Here's how the part is built. I have some questions about the finished solid (model axes, mm). A direction names the side the tool comes from. Round coordinates to 2 decimals unless told otherwise and drop trailing zeros. Loops run counter-clockwise (first coordinate to the right, second up) from the corner with the lowest first, then second, coordinate; pieces in that order, holes last. Notation, with made-up numbers: M 75,58 L 84,58 A22 ccw 84,95 Z; hole C 72,29 d4. An arc over 180 degrees is marked long. Use a Markdown table: item, result.
```python
from build123d import *

# Parameters (mm, degrees)
SKETCH1_W           = 100
SKETCH1_H           = 48
BOSS_EXTRUDE1_DEPTH = 7
CUT_EXTRUDE1_REACH  = 113.144
SKETCH2_R           = 4.5
SKETCH2_R_2         = 2.2
SKETCH3_W           = 100
SKETCH3_H           = 8
BOSS_EXTRUDE2_DEPTH = 10.2
SKETCH4_R           = 6.6
CUT_EXTRUDE2_DEPTH  = 5.25
SKETCH5_R           = 2.6
CUT_EXTRUDE3_DEPTH  = 7
SKETCH7_R           = 1.5
CUT_EXTRUDE4_DEPTH  = 112.391382072
CUT_EXTRUDE5_REACH  = 114.249
SKETCH8_R           = 1.7
SKETCH9_R           = 3
CUT_EXTRUDE6_DEPTH  = 3.5
BOSS_EXTRUDE3_DEPTH = 7
CUT_EXTRUDE7_REACH  = 116.246
FILLET1_R           = 10
FILLET2_R           = 10


with BuildPart() as part:
    # Sketch1 → Boss-Extrude1 (new body)
    with BuildSketch(Plane.XY):
        with Locations((50, 24)):
            Rectangle(SKETCH1_W, SKETCH1_H)
    extrude(amount=BOSS_EXTRUDE1_DEPTH)

    # Sketch2 → Cut-Extrude1 (cut, up to next)
    with BuildSketch(Plane.XY.offset(7), mode=Mode.PRIVATE) as cut_extrude1_sk1:
        with Locations((15, 29)):
            Circle(SKETCH2_R)
    cut_extrude1_tool1 = extrude(cut_extrude1_sk1.sketch, amount=-CUT_EXTRUDE1_REACH, mode=Mode.PRIVATE) & part.part
    # Sketch2 → Cut-Extrude1 (cut, up to next)
    with BuildSketch(Plane.XY.offset(7), mode=Mode.PRIVATE) as cut_extrude1_sk2:
        with Locations((33.75, 29)):
            Circle(SKETCH2_R_2)
    cut_extrude1_tool2 = extrude(cut_extrude1_sk2.sketch, amount=-CUT_EXTRUDE1_REACH, mode=Mode.PRIVATE) & part.part
    # Sketch2 → Cut-Extrude1 (cut, up to next)
    with BuildSketch(Plane.XY.offset(7), mode=Mode.PRIVATE) as cut_extrude1_sk3:
        with Locations((55, 29)):
            Circle(SKETCH2_R_2)
    cut_extrude1_tool3 = extrude(cut_extrude1_sk3.sketch, amount=-CUT_EXTRUDE1_REACH, mode=Mode.PRIVATE) & part.part
    # Sketch2 → Cut-Extrude1 (cut, up to next)
    with BuildSketch(Plane.XY.offset(7), mode=Mode.PRIVATE) as cut_extrude1_sk4:
        with Locations((76.25, 29)):
            Circle(SKETCH2_R_2)
    cut_extrude1_tool4 = extrude(cut_extrude1_sk4.sketch, amount=-CUT_EXTRUDE1_REACH, mode=Mode.PRIVATE) & part.part
    add(cut_extrude1_tool1.solids().sort_by_distance((15, 29, 7))[0], mode=Mode.SUBTRACT)
    add(cut_extrude1_tool2.solids().sort_by_distance((33.75, 29, 7))[0], mode=Mode.SUBTRACT)
    add(cut_extrude1_tool3.solids().sort_by_distance((55, 29, 7))[0], mode=Mode.SUBTRACT)
    add(cut_extrude1_tool4.solids().sort_by_distance((76.25, 29, 7))[0], mode=Mode.SUBTRACT)

    # Sketch3 → Boss-Extrude2 (add)
    with BuildSketch(Plane(origin=(0, 0, 0), x_dir=(-1, 0, 0), z_dir=(0, 0, -1))):
        with Locations((-50, 4)):
            Rectangle(SKETCH3_W, SKETCH3_H)
    extrude(amount=BOSS_EXTRUDE2_DEPTH)

    # Sketch4 → Cut-Extrude2 (cut)
    with BuildSketch(Plane(origin=(0, 0, 0), x_dir=(-1, 0, 0), z_dir=(0, 0, -1))):
        with Locations((-76.25, 29)):
            Circle(SKETCH4_R)
        with Locations((-55, 29)):
            Circle(SKETCH4_R)
        with Locations((-33.75, 29)):
            Circle(SKETCH4_R)
        with Locations((-15, 29)):
            Circle(SKETCH4_R)
    extrude(amount=-CUT_EXTRUDE2_DEPTH, mode=Mode.SUBTRACT)

    # Sketch5 → Cut-Extrude3 (cut)
    with BuildSketch(Plane.XY.offset(7)):
        with Locations((35.000022648, 4.052132501)):
            Circle(SKETCH5_R)
        with Locations((64.999977352, 4)):
            Circle(SKETCH5_R)
    extrude(amount=-CUT_EXTRUDE3_DEPTH, mode=Mode.SUBTRACT)

    # Sketch7 → Cut-Extrude4 (cut, through all)
    with BuildSketch(Plane.XY):
        with Locations((35.000022648, 4.052132501)):
            Circle(SKETCH7_R)
        with Locations((64.999977352, 4)):
            Circle(SKETCH7_R)
    extrude(amount=-CUT_EXTRUDE4_DEPTH, mode=Mode.SUBTRACT)

    # Sketch8 → Cut-Extrude5 (cut, up to next)
    with BuildSketch(Plane.XY.offset(7), mode=Mode.PRIVATE) as cut_extrude5_sk1:
        with Locations((10, 4.052132501)):
            Circle(SKETCH8_R)
    cut_extrude5_tool1 = extrude(cut_extrude5_sk1.sketch, amount=-CUT_EXTRUDE5_REACH, mode=Mode.PRIVATE) & part.part
    # Sketch8 → Cut-Extrude5 (cut, up to next)
    with BuildSketch(Plane.XY.offset(7), mode=Mode.PRIVATE) as cut_extrude5_sk2:
        with Locations((90, 4.052132501)):
            Circle(SKETCH8_R)
    cut_extrude5_tool2 = extrude(cut_extrude5_sk2.sketch, amount=-CUT_EXTRUDE5_REACH, mode=Mode.PRIVATE) & part.part
    add(cut_extrude5_tool1.solids().sort_by_distance((10, 4.052133, 7))[0], mode=Mode.SUBTRACT)
    add(cut_extrude5_tool2.solids().sort_by_distance((90, 4.052133, 7))[0], mode=Mode.SUBTRACT)

    # Sketch9 → Cut-Extrude6 (cut)
    with BuildSketch(Plane.XY.offset(7)):
        with Locations((10, 4.052132501)):
            Circle(SKETCH9_R)
        with Locations((90, 4.052132501)):
            Circle(SKETCH9_R)
    extrude(amount=-CUT_EXTRUDE6_DEPTH, mode=Mode.SUBTRACT)

    # Sketch10 → Boss-Extrude3 (add)
    with BuildSketch(Plane.XY.offset(7)):
        with BuildLine():
            Line((23, 52.5), (58, 52.5))
            ThreePointArc((58, 52.5), (62.5, 48), (58, 43.5))
            Line((58, 43.5), (23, 43.5))
            ThreePointArc((23, 43.5), (18.5, 48), (23, 52.5))
        make_face()
        with BuildLine():
            Line((23, 49.5), (58, 49.5))
            ThreePointArc((58, 49.5), (59.5, 48), (58, 46.5))
            Line((58, 46.5), (23, 46.5))
            ThreePointArc((23, 46.5), (21.5, 48), (23, 49.5))
        make_face(mode=Mode.SUBTRACT)
    extrude(amount=-BOSS_EXTRUDE3_DEPTH)

    # Sketch11 → Cut-Extrude7 (cut, up to next)
    with BuildSketch(Plane.XY.offset(7), mode=Mode.PRIVATE) as cut_extrude7_sk1:
        with BuildLine():
            Line((23, 49.5), (58, 49.5))
            ThreePointArc((58, 49.5), (59.5, 48), (58, 46.5))
            Line((58, 46.5), (23, 46.5))
            ThreePointArc((23, 46.5), (21.5, 48), (23, 49.5))
        make_face()
    cut_extrude7_tool1 = extrude(cut_extrude7_sk1.sketch, amount=-CUT_EXTRUDE7_REACH, mode=Mode.PRIVATE) & part.part
    add(cut_extrude7_tool1.solids().sort_by_distance((40.5, 48, 7))[0], mode=Mode.SUBTRACT)

    # Fillet1
    fillet1_edges = [part.edges().sort_by_distance(p)[0] for p in [
        (0, 48, 3.5),
        (100, 48, 3.5),
    ]]
    fillet(fillet1_edges, radius=FILLET1_R)

    # Fillet2
    fillet2_edges = [part.edges().sort_by_distance(p)[0] for p in [
        (18.5, 48, 3.5),
        (62.5, 48, 3.5),
    ]]
    fillet(fillet2_edges, radius=FILLET2_R)


solid = part.part
```
Q1. Imagine slicing it at D-D, the plane z = -8.25. Please give me the cut outline in (x, y).
Return value:
| item | result |
|---|---|
| outline | M 0,0 L 100,0 L 100,8 L 0,8 Z; hole C 10,4.05 d3.4; hole C 35,4.05 d3; hole C 65,4 d3; hole C 90,4.05 d3.4 |
Q2. Imagine slicing it at B-B, the plane x = 15. Please give me the cut outline in (y, z), then the cut area to 3 significant figures.
Return value:
| item | result |
|---|---|
| outline | M 0,-10.2 L 8,-10.2 L 8,0 L 22.4,0 L 22.4,5.25 L 24.5,5.25 L 24.5,7 L 0,7 Z; M 33.5,5.25 L 35.6,5.25 L 35.6,0 L 48.32,0 L 48.32,7 L 33.5,7 Z |
| area | 335 mm^2 |
Q3. Imagine slicing it at A-A, the plane x = 55. Please give me the cut outline in (y, z), then the cut area to 3 significant figures.
Return value:
| item | result |
|---|---|
| outline | M 0,-10.2 L 8,-10.2 L 8,0 L 22.4,0 L 22.4,5.25 L 26.8,5.25 L 26.8,7 L 0,7 Z; M 31.2,5.25 L 35.6,5.25 L 35.6,0 L 46.5,0 L 46.5,7 L 31.2,7 Z; M 49.5,0 L 52.5,0 L 52.5,7 L 49.5,7 Z |
| area | 351 mm^2 |
Q4. Will these pins go through, and if not, where does the flat tip stop? P1, Ø1.8, axis at x = 9, y = 5.5, coming from the +Z side; P2, Ø2, axis at x = 65, y = 25.5, coming from the -Z side; P3, Ø8, axis at x = 73.5, z = -3.5, coming from the +Y side.
Return value:
| item | result |
|---|---|
| P1 | stops at z = 3.5 |
| P2 | stops at z = 0 |
| P3 | stops at y = 48 |
Q5. Imagine slicing it at C-C, the plane y = 29. Give the number of separate pieces and of enclosed holes in the cut face, then the cut area to 3 significant figures.
Return value:
| item | result |
|---|---|
| separate pieces | 5 |
| enclosed holes | 0 |
| area | 384 mm^2 |
Q6. I need wall thicknesses on line 1 (Y direction, x = 55, z = 3.65); line 2 (Y direction, x = 43, z = 1.75); line 3 (Y direction, x = 10, z = 6.35). Which ranges of each line are inside material? Lowest first, please. Write a range as from..to.
Return value:
| item | result |
|---|---|
| line 1 | y = 0..22.4, 35.6..46.5, 49.5..52.5 |
| line 2 | y = 0..46.5, 49.5..52.5 |
| line 3 | y = 0..1.05, 7.05..48 |
Q7. We'd pull the mould along Y, two halves only. Please class faces 5 (the cylindrical face through (48.903, 26.472, 2.588)), 6 (the flat face through (51, 36, 0)), 7 (the cylindrical face through (3.01, 45.15, 3.55)): pulls with the +Y half, pulls with the -Y half, needs draft (parallel to the pull), parting line crosses it, or undercut.
Return value:
| item | result |
|---|---|
| face 5 | undercut |
| face 6 | needs draft |
| face 7 | pulls with the +Y half |
Q8. For faces 1 (the flat face through (12, 4, 3.5)), 2 (the cylindrical face through (21.5, 48, 3.5)), 3 (the flat face through (51, 8, -5)), 4 (the flat face through (35, 31, 5.25)), which set-ups out of +Z, -Z, +X, -X, +Y, -Y let a thin tool reach every point of the face, with its end or its side?
Return value:
| item | result |
|---|---|
| face 1 | +Z |
| face 2 | +Z, -Z |
| face 3 | -Z, +X, -X, +Y |
| face 4 | -Z |
